from build123d import *

# Parameters (mm, degrees)
F1_DEPTH = 63
F2_R     = 16
F3_DEPTH = 275.001


with BuildPart() as f1:
    # F0 (on Front) → F1 (new body)
    with BuildSketch(Plane.XZ):
        with BuildLine():
            Line((-122, 125), (-122, 0))
            Line((-122, 0), (-75, 0))
            Line((-75, 0), (-75, 22))
            Line((-75, 22), (-99, 22))
            Line((-99, 22), (-99, 125))
            ThreePointArc((-99, 125), (-69.878568, 194.292857), (0, 221.979379))
            ThreePointArc((0, 221.979379), (69.878568, 194.292857), (99, 125))
            Line((99, 125), (99, 22))
            Line((99, 22), (75, 22))
            Line((75, 22), (75, 0))
            Line((75, 0), (122, 0))
            Line((122, 0), (122, 125))
            ThreePointArc((122, 125), (99.237309, 195.320023), (39.584906, 238.962164))
            ThreePointArc((39.584906, 238.962164), (33.371114, 243.508221), (31, 250.833223))
            Line((31, 250.833223), (31, 275))
            Line((31, 275), (0, 275))
            Line((0, 275), (-31, 275))
            Line((-31, 275), (-31, 250.833223))
            ThreePointArc((-31, 250.833223), (-33.371114, 243.508221), (-39.584906, 238.962164))
            ThreePointArc((-39.584906, 238.962164), (-99.237309, 195.320023), (-122, 125))
        make_face()
    extrude(amount=F1_DEPTH)

    # F2 (on face) → F3 (cut, through all)
    with BuildSketch(Plane.XY.offset(275)):
        with Locations((0, -31.5)):
            Circle(F2_R)
    extrude(amount=-F3_DEPTH, mode=Mode.SUBTRACT)


solid = f1.part
Geometry check sheet. Reference: the model listing, model coordinates, mm. A direction names the side the tool comes from. Give positions to 0.01 mm unless a question says otherwise; leave off trailing zeros. Order: outer loops, then holes, each group sorted by start corner. A loop starts at its lowest first (then second) coordinate and runs counter-clockwise, first axis right, second up.
1) Tool access check on faces 1 (the flat face through (75, -31, 11)), 2 (the flat face through (31, -31, 263)), 3 (the flat face through (-122, -31, 63)), 4 (the cylindrical face through (69.102, -31.059, 195.045)). Record the directions out of +Z, -Z, +X, -X, +Y, -Y that give a thin tool (end or side, any length) a straight path to the whole face; none if there is none.
Results are:
face 1: -Z, +Y, -Y
face 2: +Z, +X, +Y, -Y
face 3: +Z, -Z, -X, +Y, -Y
face 4: +Y, -Y
2) Material ranges on probe 1 along X at (y, z) = (-31.5, 259.5); probe 2 along Y at (x, z) = (0, 253.5); probe 3 along X at (y, z) = (-16.5, 107), recorded low to high.
Results are:
probe 1: x = -31 to -16, 16 to 31
probe 2: y = -63 to -47.5, -15.5 to 0
probe 3: x = -122 to -99, 99 to 122
3) Cross-section at B-B (y = -31.5). Record the boundary of the cut face in (x, z), then the cut area to 3 significant figures.
Results are:
outline: (-122, 0) - (-75, 0) - (-75, 22) - (-99, 22) - (-99, 125) arc R97 cw to (-16, 220.98) - (-16, 275) - (-31, 275) - (-31, 250.83) arc R12.5 cw to (-39.58, 238.96) arc R120 ccw to (-122, 125) - close; (16, 220.98) arc R97 cw to (99, 125) - (99, 22) - (75, 22) - (75, 0) - (122, 0) - (122, 125) arc R120 ccw to (39.58, 238.96) arc R12.5 cw to (31, 250.83) - (31, 275) - (16, 275) - close
area: 15,000 mm2
4) Gauge pin test, flat ends, axial feed: pin 1 (7.5 mm diameter, centred on y = -17, z = 266.5, fed in from +X); pin 2 (1 mm diameter, centred on y = -45.5, z = 228.5, fed in from -X); pin 3 (1.5 mm diameter, centred on x = -27.5, y = -23.5, fed in from -Z). Record the tip position at first contact, or that the pin passes through.
Results are:
pin 1: stops at x = 31
pin 2: stops at x = -63.57
pin 3: stops at z = 218.38
5) Cross-section at A-A (z = 67.5). Record the boundary of the cut face in (x, y), then the cut area to 3 significant figures.
Results are:
outline: (-122, -63) - (-99, -63) - (-99, 0) - (-122, 0) - close; (99, -63) - (122, -63) - (122, 0) - (99, 0) - close
area: 2,900 mm2
6) Draft check along Y on faces 5 (the flat face through (-28, -63, 220)), 6 (the flat face through (-31, -31, 263)), 7 (the cylindrical face through (-3.47, -47.12, 248.37)). Enter one of: released by +Y, released by -Y, zero draft, split by the parting line, or undercut.
Results are:
face 5: released by -Y
face 6: zero draft
face 7: undercut
7) Cross-section at C-C (x = 13). Record the boundary of the cut face in (y, z), then the cut area to 3 significant figures.
Results are:
outline: (-63, 221.37) - (-40.83, 221.37) - (-40.83, 275) - (-63, 275) - close; (-22.17, 221.37) - (0, 221.37) - (0, 275) - (-22.17, 275) - close
area: 2,380 mm2
8) Cross-section at D-D (y = -51). Record the boundary of the cut face in (x, z).
Results are:
outline: (-122, 0) - (-75, 0) - (-75, 22) - (-99, 22) - (-99, 125) arc R97 cw to (0, 221.98) arc R97 cw to (99, 125) - (99, 22) - (75, 22) - (75, 0) - (122, 0) - (122, 125) arc R120 ccw to (39.58, 238.96) arc R12.5 cw to (31, 250.83) - (31, 275) - (-31, 275) - (-31, 250.83) arc R12.5 cw to (-39.58, 238.96) arc R120 ccw to (-122, 125) - close
